from build123d import *

# Parameters (mm, degrees)
RESSALTO_EXTRUS_O2_DEPTH = 30
CASCA1_T                 = -2
RESSALTO_EXTRUS_O3_DEPTH = 28
RESSALTO_EXTRUS_O4_DEPTH = 13
CASCA2_START             = 2
CASCA2_DEPTH             = 13
RESSALTO_EXTRUS_O5_DEPTH = 13
RESSALTO_EXTRUS_O6_DEPTH = 13
CORTE_EXTRUS_O1_DEPTH    = 60
RESSALTO_EXTRUS_O7_DEPTH = 1
RESSALTO_EXTRUS_O8_START = -1
RESSALTO_EXTRUS_O8_DEPTH = 1
ESBO_O16_R               = 11
CORTE_EXTRUS_O2_DEPTH    = 60
ESBO_O17_R               = 2.5
CORTE_EXTRUS_O3_DEPTH    = 15
FILETE1_R                = 1
ESBO_O18_W               = 1
ESBO_O18_H               = 2
RESSALTO_EXTRUS_O9_DEPTH = 6


# Read off the part's stored shape, not the designer's step: Casca2, Ressalto-extrusão5, Ressalto-extrusão6
with BuildPart() as part:
    # Esboço2 → Ressalto-extrusão2 (new body)
    with BuildSketch(Plane(origin=(0, 0, 0), x_dir=(1, 0, 0), z_dir=(0, 1, 0))):
        with BuildLine():
            Line((-30, 35), (-30, -35))
            ThreePointArc((-30, -35), (0, -28), (30, -35))
            Line((30, -35), (30, 35))
            ThreePointArc((30, 35), (0, 28), (-30, 35))
        make_face()
    extrude(amount=RESSALTO_EXTRUS_O2_DEPTH)

    # Casca1
    casca1_openings = [part.faces().sort_by_distance(p)[0] for p in [
        (0, 30, 0),
    ]]
    offset(amount=CASCA1_T, openings=casca1_openings, kind=Kind.INTERSECTION)

    # Esboço5 → Ressalto-extrusão3 (add)
    with BuildSketch(Plane(origin=(0, 2, 0), x_dir=(1, 0, 0), z_dir=(0, 1, 0))):
        with BuildLine():
            Line((28, 22.89910018), (28, 24.89910018))
            Line((28, 24.89910018), (23, 24.89910018))
            Line((23, 24.89910018), (23, 29.89910018))
            ThreePointArc((23, 29.89910018), (22.002508446, 29.559318185), (21, 29.234636771))
            Line((21, 29.234636771), (21, 22.89910018))
            Line((21, 22.89910018), (28, 22.89910018))
        make_face()
        with BuildLine():
            ThreePointArc((-23, -29.89910018), (-22.002508446, -29.559318185), (-21, -29.234636771))
            Line((-21, -29.234636771), (-21, -22.89910018))
            Line((-21, -22.89910018), (-28, -22.89910018))
            Line((-28, -22.89910018), (-28, -24.89910018))
            Line((-28, -24.89910018), (-23, -24.89910018))
            Line((-23, -24.89910018), (-23, -29.89910018))
        make_face()
        with BuildLine():
            Line((-21, 22.89910018), (-21, 29.234636771))
            ThreePointArc((-21, 29.234636771), (-22.002508446, 29.559318185), (-23, 29.89910018))
            Line((-23, 29.89910018), (-23, 24.89910018))
            Line((-23, 24.89910018), (-28, 24.89910018))
            Line((-28, 24.89910018), (-28, 22.89910018))
            Line((-28, 22.89910018), (-21, 22.89910018))
        make_face()
        with BuildLine():
            Line((28, -24.89910018), (28, -22.89910018))
            Line((28, -22.89910018), (21, -22.89910018))
            Line((21, -22.89910018), (21, -29.234636771))
            ThreePointArc((21, -29.234636771), (22.002508446, -29.559318185), (23, -29.89910018))
            Line((23, -29.89910018), (23, -24.89910018))
            Line((23, -24.89910018), (28, -24.89910018))
        make_face()
    extrude(amount=RESSALTO_EXTRUS_O3_DEPTH)

    # Esboço6 → Ressalto-extrusão4 (add)
    with BuildSketch(Plane(origin=(0, 2, 0), x_dir=(1, 0, 0), z_dir=(0, 1, 0))):
        with BuildLine():
            Line((-15.5, 27.743110585), (-15.5, -27.743110585))
            ThreePointArc((-15.5, -27.743110585), (0, -26), (15.5, -27.743110585))
            Line((15.5, -27.743110585), (15.5, 27.743110585))
            ThreePointArc((15.5, 27.743110585), (0, 26), (-15.5, 27.743110585))
        make_face()
    extrude(amount=RESSALTO_EXTRUS_O4_DEPTH)

    # Casca2 outline → Casca2 (cut)
    with BuildSketch(Plane(origin=(0, 0, 0), x_dir=(1, 0, 0), z_dir=(0, 1, 0)).offset(CASCA2_START)):
        with BuildLine():
            Line((-13.5, 27.318233549), (-13.5, -27.318233549))
            ThreePointArc((-13.5, -27.318233549), (0, -26), (13.5, -27.318233549))
            Line((13.5, -27.318233549), (13.5, 27.318233549))
            ThreePointArc((13.5, 27.318233549), (0, 26), (-13.5, 27.318233549))
        make_face()
    extrude(amount=CASCA2_DEPTH, mode=Mode.SUBTRACT)

    # Ressalto-extrusão5 outline → Ressalto-extrusão5 (add)
    with BuildSketch(Plane(origin=(0, 2, 0), x_dir=(1, 0, 0), z_dir=(0, 1, 0))):
        with BuildLine():
            Line((15.5, 27.743110585), (15.5, -27.743110585))
            ThreePointArc((15.5, -27.743110585), (18.265230976, -28.432709484), (21, -29.234636771))
            Line((21, -29.234636771), (21, -22.89910018))
            Line((21, -22.89910018), (28, -22.89910018))
            Line((28, -22.89910018), (28, 22.89910018))
            Line((28, 22.89910018), (21, 22.89910018))
            Line((21, 22.89910018), (21, 29.234636771))
            ThreePointArc((21, 29.234636771), (18.265230976, 28.432709484), (15.5, 27.743110585))
        make_face()
    extrude(amount=RESSALTO_EXTRUS_O5_DEPTH)

    # Ressalto-extrusão6 outline → Ressalto-extrusão6 (add)
    with BuildSketch(Plane(origin=(0, 2, 0), x_dir=(1, 0, 0), z_dir=(0, 1, 0))):
        with BuildLine():
            Line((-21, -22.89910018), (-21, -29.234636771))
            ThreePointArc((-21, -29.234636771), (-18.265230976, -28.432709484), (-15.5, -27.743110585))
            Line((-15.5, -27.743110585), (-15.5, 27.743110585))
            ThreePointArc((-15.5, 27.743110585), (-18.265230976, 28.432709484), (-21, 29.234636771))
            Line((-21, 29.234636771), (-21, 22.89910018))
            Line((-21, 22.89910018), (-28, 22.89910018))
            Line((-28, 22.89910018), (-28, -22.89910018))
            Line((-28, -22.89910018), (-21, -22.89910018))
        make_face()
    extrude(amount=RESSALTO_EXTRUS_O6_DEPTH)

    # Esboço9 → Corte-extrusão1 (cut)
    with BuildSketch(Plane.ZY.offset(30)):
        with BuildLine():
            ThreePointArc((-11.532562595, 30), (-12.62781283, 27.088420816), (-13, 24))
            ThreePointArc((-13, 24), (0, 11), (13, 24))
            ThreePointArc((13, 24), (12.62781283, 27.088420816), (11.532562595, 30))
            Line((11.532562595, 30), (-11.532562595, 30))
        make_face()
        with BuildLine():
            ThreePointArc((11.532562595, 30), (0, 37), (-11.532562595, 30))
            Line((-11.532562595, 30), (11.532562595, 30))
        make_face()
        with BuildLine():
            Line((-13, 44), (-13, 30))
            Line((-13, 30), (-11.532562595, 30))
            ThreePointArc((-11.532562595, 30), (0, 37), (11.532562595, 30))
            Line((11.532562595, 30), (13, 30))
            Line((13, 30), (13, 44))
            Line((13, 44), (-13, 44))
        make_face()
        with BuildLine():
            ThreePointArc((11.532562595, 30), (12.62781283, 27.088420816), (13, 24))
            Line((13, 24), (13, 30))
            Line((13, 30), (11.532562595, 30))
        make_face()
        with BuildLine():
            Line((-13, 30), (-13, 24))
            ThreePointArc((-13, 24), (-12.62781283, 27.088420816), (-11.532562595, 30))
            Line((-11.532562595, 30), (-13, 30))
        make_face()
    extrude(amount=-CORTE_EXTRUS_O1_DEPTH, mode=Mode.SUBTRACT)

    # Esboço14 → Ressalto-extrusão7 (add)
    with BuildSketch(Plane.ZY.offset(30)):
        with BuildLine():
            Line((-13, 24), (13, 24))
            ThreePointArc((13, 24), (0, 11), (-13, 24))
        make_face()
    extrude(amount=-RESSALTO_EXTRUS_O7_DEPTH)

    # Esboço15 → Ressalto-extrusão8 (add)
    with BuildSketch(Plane(origin=(30, 0, 0), x_dir=(0, 0, -1), z_dir=(1, 0, 0)).offset(RESSALTO_EXTRUS_O8_START)):
        with BuildLine():
            Line((-13, 24), (13, 24))
            ThreePointArc((13, 24), (0, 11), (-13, 24))
        make_face()
    extrude(amount=RESSALTO_EXTRUS_O8_DEPTH)

    # Esboço16 → Corte-extrusão2 (cut)
    with BuildSketch(Plane.ZY.offset(30)):
        with Locations((0, 24)):
            Circle(ESBO_O16_R)
    extrude(amount=-CORTE_EXTRUS_O2_DEPTH, mode=Mode.SUBTRACT)

    # Esboço17 → Corte-extrusão3 (cut)
    with BuildSketch(Plane(origin=(0, 15, 0), x_dir=(1, 0, 0), z_dir=(0, 1, 0))):
        with Locations(Location((18, 17, 0), (0, 0, 270))):
            Circle(ESBO_O17_R)
        with Locations(Location((-18, -17, 0), (0, 0, 270))):
            Circle(ESBO_O17_R)
        with Locations(Location((18, -17, 0), (0, 0, 270))):
            Circle(ESBO_O17_R)
        with Locations(Location((-18, 17, 0), (0, 0, 270))):
            Circle(ESBO_O17_R)
    extrude(amount=-CORTE_EXTRUS_O3_DEPTH, mode=Mode.SUBTRACT)

    # Filete1
    filete1_edges = [part.edges().sort_by_distance(p)[0] for p in [
        (-30, 15, 35),
        (-30, 15, -35),
        (30, 15, -35),
        (30, 15, 35),
    ]]
    fillet(filete1_edges, radius=FILETE1_R)

    # Esboço18 → Ressalto-extrusão9 (add)
    with BuildSketch(Plane(origin=(0, 24, 0), x_dir=(1, 0, 0), z_dir=(0, 1, 0))):
        with Locations((-29.5, 12)):
            Rectangle(ESBO_O18_W, ESBO_O18_H)
        with Locations((-29.5, -12)):
            Rectangle(ESBO_O18_W, ESBO_O18_H)
        with Locations((29.5, 12)):
            Rectangle(ESBO_O18_W, ESBO_O18_H)
        with Locations((29.5, -12)):
            Rectangle(ESBO_O18_W, ESBO_O18_H)
    extrude(amount=RESSALTO_EXTRUS_O9_DEPTH)


solid = part.part
Check sheet for the modelled part. Datum: model origin and axes. Units: mm. A direction names the side the tool comes from. Give positions to 0.01 mm unless a question says otherwise; leave off trailing zeros. Loops run counter-clockwise (first coordinate to the right, second up) from the corner with the lowest first, then second, coordinate; pieces in that order, holes last. Notation, with made-up numbers: M -21,21 L 33,21 A22 ccw 33,47 Z; hole C 14.5,85.5 d5. An arc over 180 degrees is marked long. Return JSON: item names as keys, results as strings. Group by question number.
1. Tool access check on faces 5 (the flat face through (-25, 22, -22.899)), 6 (the cylindrical face through (0, 15, 28)). Record the directions out of +Z, -Z, +X, -X, +Y, -Y that give a thin tool (end or side, any length) a straight path to the whole face; none if there is none.
2. Cross-section at D-D on z = 0. Record the boundary of the cut face in (x, y).
3. Cross-section at B-B on x = -18. Record the boundary of the cut face in (y, z).
4. Cross-section at A-A on z = -17. Record the boundary of the cut face in (x, y).
5. Cross-section at C-C on y = 19.75. State how many separate pieces and enclosed holes the cut face has, plus the area to 3 significant figures.
6. Go/stop test with flat-tipped pins: pin 1 (2.5 mm diameter, centred on x = -25.5, z = -28, fed in from +Y); pin 2 (0.5 mm diameter, centred on x = -29.5, y = 28, fed in from +Z); pin 3 (16 mm diameter, centred on x = -20.5, z = -21, fed in from +Y); pin 4 (1.5 mm diameter, centred on x = 24.5, y = 14.5, fed in from +Z). Record where each tip stops, or that it passes through.
7. Thickness scan on L1, parallel to X at y = 7.5, z = -17; L2, parallel to X at y = 28.75, z = -19; L3, parallel to Z at x = 22.5, y = 19.25. Record the ranges inside material, lowest first.
8. Mould release check, pull along X, two halves, no side actions. Record for faces 1 (the flat face through (24, 22, -22.899)), 2 (the flat face through (25, 16, 24.899)), 3 (the flat face through (-0.1, 30, -26.2)), 4 (the flat face through (30, 12, 0)): released by +X, released by -X, zero draft, split by the parting line, or undercut.
Return value:
{
 "1": {"face 5": "+Y", "face 6": "+Z, +Y, -Y"},
 "2": {"outline": "M -30,0 L 30,0 L 30,13 L 29,13 L 29,11 L 13.5,11 L 13.5,2 L -13.5,2 L -13.5,11 L -29,11 L -29,13 L -30,13 Z"},
 "3": {"outline": "M 0,-30.43 L 30,-30.43 L 30,-28.36 L 15,-28.36 L 15,-19.5 L 0,-19.5 Z; M 0,-14.5 L 15,-14.5 L 15,-9.38 A13 cw 15,9.38 L 15,14.5 L 0,14.5 Z; M 0,19.5 L 15,19.5 L 15,28.36 L 30,28.36 L 30,30.43 L 0,30.43 Z"},
 "4": {"outline": "M -30,0 L -20.5,0 L -20.5,15 L -28,15 L -28,30 L -30,30 Z; M -15.5,0 L 15.5,0 L 15.5,15 L 13.5,15 L 13.5,2 L -13.5,2 L -13.5,15 L -15.5,15 Z; M 20.5,0 L 30,0 L 30,30 L 28,30 L 28,15 L 20.5,15 Z"},
 "5": {"separate pieces": "2", "enclosed holes": "4", "area": "508 mm^2"},
 "6": {"pin 1": "y = 2", "pin 2": "z = 34.38", "pin 3": "y = 30", "pin 4": "z = 32.88"},
 "7": {"L1": "-30 to -20.5, -15.5 to -13.5, 13.5 to 15.5, 20.5 to 30", "L2": "-30 to -28, 28 to 30", "L3": "-31.84 to -22.9, 22.9 to 31.84"},
 "8": {"face 1": "undercut", "face 2": "undercut", "face 3": "zero draft", "face 4": "released by +X"}
}
